The listing builds one solid part. Answer for the finished solid, in the listing's coordinates (mm). A direction names the side the tool comes from. Coordinates: 2 decimals unless noted, no trailing zeros. Loops run counter-clockwise (first coordinate to the right, second up) from the corner with the lowest first, then second, coordinate; pieces in that order, holes last. Notation, with made-up numbers: (-18, -9.5) - (6, -9.5) arc R27 ccw to (6, 26.5) - close; hole circle Ø9 at (-38.75, 6.25). An arc over 180 degrees is marked (long way). One line per question, with ' | ' between items.
from build123d import *

# Parameters (mm, degrees)
SKETCH_1_R                  = 7.5
SKETCH_1_R_2                = 6
EXTRUDE_1_DEPTH             = 17
CUT_EXTRUDE_1_REACH         = 25.88
CUT_EXTRUDE_1_END_RADIUS    = 6
SKETCH_2_W                  = 1
SKETCH_2_H                  = 17
SKETCH_3_W                  = 4
SKETCH_3_H                  = 17
EXTRUDE_2_DEPTH             = 5
EXTRUDE_2_DIRECTION_2_REACH = 25.88
CUT_EXTRUDE_START           = -2
CUT_EXTRUDE_4_DEPTH         = 2
CUT_EXTRUDE_2_REACH         = 26.274
SKETCH_4_R                  = 1.25
CUT_EXTRUDE_3_DEPTH         = 1.5


with BuildPart() as part:
    # 草图1 → 凸台-拉伸1 (new body)
    with BuildSketch(Plane(origin=(0, 0, 0), x_dir=(1, 0, 0), z_dir=(0, 1, 0))):
        with Locations(Location((0, 0, 0), (0, 0, 270))):
            Circle(SKETCH_1_R)
        with Locations(Location((0, 0, 0), (0, 0, 270))):
            Circle(SKETCH_1_R_2, mode=Mode.SUBTRACT)
    extrude(amount=EXTRUDE_1_DEPTH)

    # 切除-拉伸1: up to this cylinder (the profile starts outside it)
    cut_extrude_1_end = Plane(origin=(0, 8.5, 0), z_dir=(0, -1, 0)) * Cylinder(CUT_EXTRUDE_1_END_RADIUS, 64.76, mode=Mode.PRIVATE)
    # 草图2 → 切除-拉伸1 (cut, up to the surface)
    with BuildSketch(Plane.XY.offset(7.5), mode=Mode.PRIVATE) as cut_extrude_1_sk1:
        with Locations((0, 8.5)):
            Rectangle(SKETCH_2_W, SKETCH_2_H)
    cut_extrude_1_tool1 = extrude(cut_extrude_1_sk1.sketch, amount=-CUT_EXTRUDE_1_REACH, mode=Mode.PRIVATE) - cut_extrude_1_end
    add(cut_extrude_1_tool1.solids().sort_by_distance((0, 8.5, 7.5))[0], mode=Mode.SUBTRACT)

    # 草图3 → 凸台-拉伸2 (add)
    with BuildSketch(Plane.XY.offset(7.5)):
        with Locations((-2.5, 8.5)):
            Rectangle(SKETCH_3_W, SKETCH_3_H)
        with Locations((2.5, 8.5)):
            Rectangle(SKETCH_3_W, SKETCH_3_H)
    extrude(amount=EXTRUDE_2_DEPTH)

    # 草图3 → 凸台-拉伸2 direction 2 (add, up to next)
    with BuildSketch(Plane.XY.offset(7.5), mode=Mode.PRIVATE) as extrude_2_direction_2_sk1:
        with Locations((-2.5, 8.5)):
            Rectangle(SKETCH_3_W, SKETCH_3_H)
    extrude_2_direction_2_tool1 = extrude(extrude_2_direction_2_sk1.sketch, amount=-EXTRUDE_2_DIRECTION_2_REACH, mode=Mode.PRIVATE) - part.part
    # 草图3 → 凸台-拉伸2 direction 2 (add, up to next)
    with BuildSketch(Plane.XY.offset(7.5), mode=Mode.PRIVATE) as extrude_2_direction_2_sk2:
        with Locations((2.5, 8.5)):
            Rectangle(SKETCH_3_W, SKETCH_3_H)
    extrude_2_direction_2_tool2 = extrude(extrude_2_direction_2_sk2.sketch, amount=-EXTRUDE_2_DIRECTION_2_REACH, mode=Mode.PRIVATE) - part.part
    add(extrude_2_direction_2_tool1.solids().sort_by_distance((-2.5, 8.5, 7.5))[0])
    add(extrude_2_direction_2_tool2.solids().sort_by_distance((2.5, 8.5, 7.5))[0])

    # 草图7 → 切除-拉伸4 (cut)
    with BuildSketch(Plane(origin=(0, 17, 0), x_dir=(1, 0, 0), z_dir=(0, 1, 0)).offset(CUT_EXTRUDE_START)):
        with BuildLine():
            Line((-4.5, -6), (-4.5, -12.5))
            Line((-4.5, -12.5), (4.5, -12.5))
            Line((4.5, -12.5), (4.5, -6))
            ThreePointArc((4.5, -6), (0, -7.5), (-4.5, -6))
        make_face()
    extrude(amount=CUT_EXTRUDE_4_DEPTH, mode=Mode.SUBTRACT)

    # 切除-拉伸2: up to this face of the body (flat: up to its plane)
    cut_extrude_2_end = Plane(part.part.faces().sort_by_distance((4.5, 7.5, 9.25))[0])
    # 草图4 → 切除-拉伸2 (cut, up to the picked face)
    with BuildSketch(Plane.ZY.offset(4.5), mode=Mode.PRIVATE) as cut_extrude_2_sk1:
        with Locations(Location((9.25, 11.5, 0), (0, 0, 270))):
            Circle(SKETCH_4_R)
    cut_extrude_2_tool1 = split(extrude(cut_extrude_2_sk1.sketch, amount=-CUT_EXTRUDE_2_REACH, mode=Mode.PRIVATE), bisect_by=cut_extrude_2_end, keep=Keep.BOTH, mode=Mode.PRIVATE)
    # 草图4 → 切除-拉伸2 (cut, up to the picked face)
    with BuildSketch(Plane.ZY.offset(4.5), mode=Mode.PRIVATE) as cut_extrude_2_sk2:
        with Locations(Location((9.25, 3.5, 0), (0, 0, 270))):
            Circle(SKETCH_4_R)
    cut_extrude_2_tool2 = split(extrude(cut_extrude_2_sk2.sketch, amount=-CUT_EXTRUDE_2_REACH, mode=Mode.PRIVATE), bisect_by=cut_extrude_2_end, keep=Keep.BOTH, mode=Mode.PRIVATE)
    add(cut_extrude_2_tool1.solids().sort_by(Axis((-4.5, 11.5, 9.25), (1, 0, 0)))[0], mode=Mode.SUBTRACT)
    add(cut_extrude_2_tool2.solids().sort_by(Axis((-4.5, 3.5, 9.25), (1, 0, 0)))[0], mode=Mode.SUBTRACT)

    # 草图5 → 切除-拉伸3 (cut)
    with BuildSketch(Plane(origin=(4.5, 0, 0), x_dir=(0, 0, -1), z_dir=(1, 0, 0))):
        Polygon((-9.25, 9.190598923), (-7.25, 10.345299462), (-7.25, 12.654700538), (-9.25, 13.809401077), (-11.25, 12.654700538), (-11.25, 10.345299462), align=None)
        Polygon((-9.25, 1.190598923), (-7.25, 2.345299462), (-7.25, 4.654700538), (-9.25, 5.809401077), (-11.25, 4.654700538), (-11.25, 2.345299462), align=None)
    extrude(amount=-CUT_EXTRUDE_3_DEPTH, mode=Mode.SUBTRACT)


solid = part.part
Item 1: Find the intervals of material crossed by line 1 (X direction, y = 8.25, z = 8.75); line 2 (X direction, y = 8.25, z = 0); line 3 (Z direction, x = 1.25, y = 3.25), in increasing order. Write a range as [from, to].
Taken from the geometry:
line 1: x = [-4.5, -0.5], [0.5, 4.5] | line 2: x = [-7.5, -6], [6, 7.5] | line 3: z = [-7.4, -5.87], [5.87, 8.03], [10.47, 12.5]
Item 2: Find section A-A, the plane y = 11.5. Write down the section's boundary in (x, z).
Taken from the geometry:
outline: (-4.5, 6) arc R7.5 ccw (long way) to (4.5, 6) - (4.5, 7.25) - (3, 7.25) - (3, 8) - (0.5, 8) - (0.5, 5.98) arc R6 cw (long way) to (-0.5, 5.98) - (-0.5, 8) - (-4.5, 8) - close; (-4.5, 10.5) - (-0.5, 10.5) - (-0.5, 12.5) - (-4.5, 12.5) - close; (0.5, 10.5) - (3, 10.5) - (3, 11.25) - (4.5, 11.25) - (4.5, 12.5) - (0.5, 12.5) - close
Item 3: Each of these flat-tipped pins is pushed along its axis until it touches: pin 1 Ø2 at (x, z) = (-2.5, -2) entering from -Y; pin 2 Ø3 at (y, z) = (3.5, 9.25) entering from -X; pin 3 Ø2 at (y, z) = (3.5, 8.5) entering from +X; pin 4 Ø1.2 at (x, y) = (4, 11.5) entering from -Z. Where does it stop, or does it pass through?
Taken from the geometry:
pin 1: passes through | pin 2: stops at x = -4.5 | pin 3: stops at x = 3 | pin 4: stops at z = -6.69
Item 4: Find section C-C, the plane z = 0. Write down the section's boundary in (x, y).
Taken from the geometry:
outline: (-7.5, 0) - (-6, 0) - (-6, 17) - (-7.5, 17) - close; (6, 0) - (7.5, 0) - (7.5, 17) - (6, 17) - close
Item 5: Which of the six approach directions +Z, -Z, +X, -X, +Y, -Y give full straight-line access (tool end or side, diameter ignored) to faces 5 (the face through (-0.5, 8, 9)), 6 (the face through (3, 12, 11)), 7 (the face through (-4.5, 7, 9)), 8 (the face through (1.732, 12.421, 10.095))?
Taken from the geometry:
face 5: +Z, +Y, -Y | face 6: +X | face 7: +Z, -X, +Y, -Y | face 8: +X, -X
Item 6: Find section B-B, the plane x = -1.25. Write down the section's boundary in (y, z).
Taken from the geometry:
outline: (0, -7.4) - (17, -7.4) - (17, -5.87) - (0, -5.87) - close; (0, 5.87) - (17, 5.87) - (17, 7.4) - (15, 7.4) - (15, 12.5) - (0, 12.5) - close; hole circle Ø2.5 at (3.5, 9.25); hole circle Ø2.5 at (11.5, 9.25)
Item 7: The mould has two halves that part along Y. Classify faces 1 (the face through (1.1, 0, 6.3)), 2 (the face through (-3, 15, 10)), 3 (the face through (4, 12, 11.25)), 4 (the face through (2, 8, 12.5)): pulls with the +Y half, pulls with the -Y half, needs draft (parallel to the pull), parting line crosses it, or undercut.
Taken from the geometry:
face 1: pulls with the -Y half | face 2: pulls with the +Y half | face 3: undercut | face 4: needs draft
Item 8: Find section D-D, the plane x = 3.75. Write down the section's boundary in (y, z).
Taken from the geometry:
outline: (0, -6.5) - (17, -6.5) - (17, -4.68) - (0, -4.68) - close; (0, 4.68) - (17, 4.68) - (17, 6.5) - (15, 6.5) - (15, 12.5) - (0, 12.5) - close; hole (1.19, 9.25) - (2.35, 7.25) - (4.65, 7.25) - (5.81, 9.25) - (4.65, 11.25) - (2.35, 11.25) - close; hole (9.19, 9.25) - (10.35, 7.25) - (12.65, 7.25) - (13.81, 9.25) - (12.65, 11.25) - (10.35, 11.25) - close
